For this review, use the dimensioned drawing (mm, ordinates from the lowest corner) and the shaded views. A direction names the side the tool comes from. Give positions to 0.01 mm unless a question says otherwise; leave off trailing zeros. Write each loop counter-clockwise with the first axis right and the second up, starting at its lowest first coordinate (ties: lowest second). Pieces come first, ordered by that corner, then holes. Notation, with made-up numbers: M -9.75,26.25 L 30.25,26.25 A31 cw 30.25,53.25 Z; hole C 8.5,53.5 d11. An arc over 180 degrees is marked long. Answer in a Markdown table with one row per item.
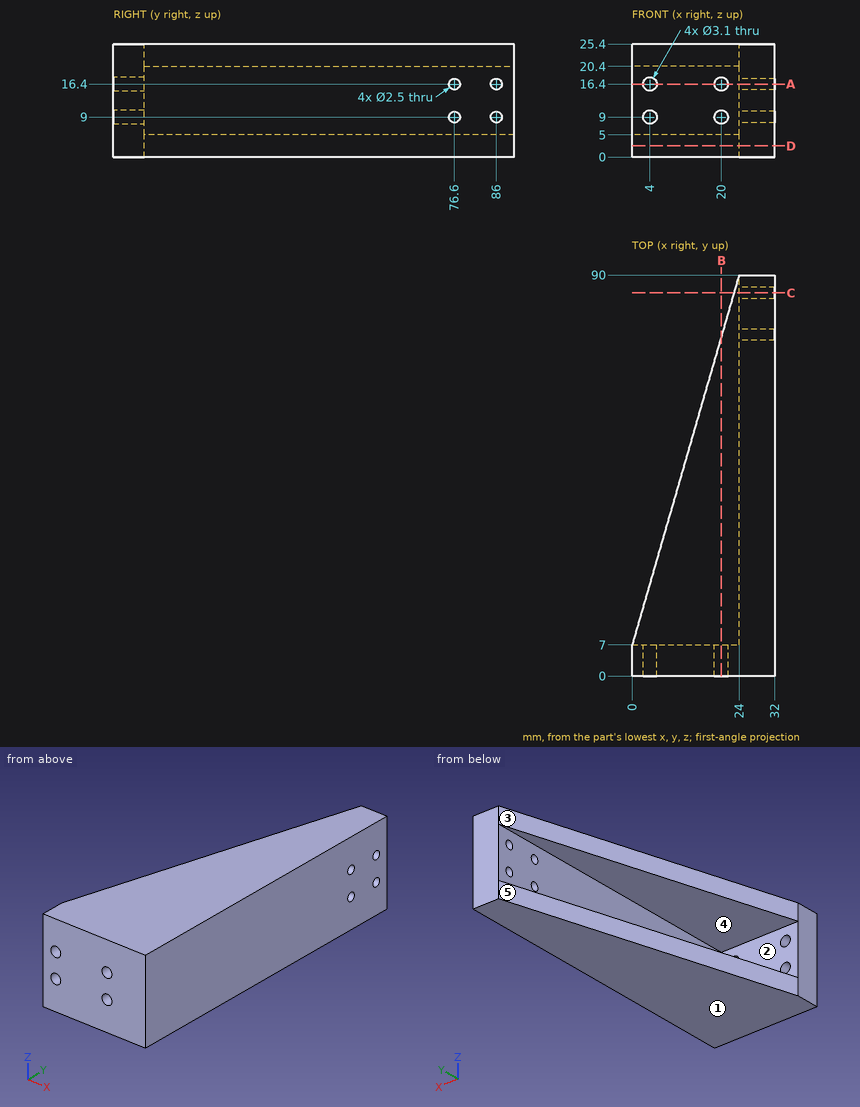
1) Add section A-A (z = 16.4). Write out the cut boundary in (x, y).
Geometry says:
| item | result |
|---|---|
| outline | M 0,0 L 2.45,0 L 2.45,7 L 0,7 Z; M 5.55,0 L 18.45,0 L 18.45,7 L 5.55,7 Z; M 21.55,0 L 32,0 L 32,75.35 L 24,75.35 L 24,7 L 21.55,7 Z; M 24,77.85 L 32,77.85 L 32,84.75 L 24,84.75 Z; M 24,87.25 L 32,87.25 L 32,90 L 24,90 Z |
2) The part is to be moulded in two halves that separate along Z. For the marked faces 1, 2 and 3, say which applies: released by +Z, released by -Z, zero draft, split by the parting line, or undercut.
Geometry says:
| item | result |
|---|---|
| face 1 | released by -Z |
| face 2 | undercut |
| face 3 | zero draft |
3) Add section B-B (x = 20). Write out the cut boundary in (y, z), and give its area (3 significant figures).
Geometry says:
| item | result |
|---|---|
| outline | M 0,0 L 76.17,0 L 76.17,5 L 7,5 L 7,7.45 L 0,7.45 Z; M 0,10.55 L 7,10.55 L 7,14.85 L 0,14.85 Z; M 0,17.95 L 7,17.95 L 7,20.4 L 76.17,20.4 L 76.17,25.4 L 0,25.4 Z |
| area | 826 mm^2 |
4) Add section D-D (z = 2.5). Write out the cut boundary in (x, y), and give its area (3 significant figures).
Geometry says:
| item | result |
|---|---|
| outline | M 0,0 L 32,0 L 32,90 L 24,90 L 0,7 Z |
| area | 1,880 mm^2 |
5) To check wall thickness, follow probe 1 along Y at (x, z) = (27.25, 9); probe 2 along Y at (x, z) = (26, 9.5); probe 3 along Z at (x, y) = (13, 23). State the ranges of each line that lie inside material, in increasing order. Write a range as [from, to].
Geometry says:
| item | result |
|---|---|
| probe 1 | [0, 75.35], [77.85, 84.75], [87.25, 90] |
| probe 2 | [0, 75.45], [77.75, 84.85], [87.15, 90] |
| probe 3 | [0, 5], [20.4, 25.4] |
6) For the marked faces 4 and 5, list the 3-axis set-ups (+Z, -Z, +X, -X, +Y, -Y) from which the entire face can be reached by the end or side of a thin tool; tool diameter is ignored.
Geometry says:
| item | result |
|---|---|
| face 4 | -X, +Y |
| face 5 | +Z, -Z, -X, +Y |
7) Insertion check: P1, Ø5, axis at x = 20.5, z = 10.5, coming from the +Y side; P2, Ø4, axis at y = 76.6, z = 16.4, coming from the -X side; P3, Ø2, axis at y = 86, z = 9, coming from the +X side; P4, Ø10, axis at y = 22, z = 7, coming from the -X side. Each pin has a flat end and moves straight along its axis. Give the tip position at first contact, or say it passes through.
Geometry says:
| item | result |
|---|---|
| P1 | y = 7 |
| P2 | x = 24 |
| P3 | through |
| P4 | x = 3.01 |
8) Add section C-C (y = 86). Write out the cut boundary in (x, z).
Geometry says:
| item | result |
|---|---|
| outline | M 22.84,0 L 32,0 L 32,7.75 L 24,7.75 L 24,5 L 22.84,5 Z; M 22.84,20.4 L 24,20.4 L 24,17.65 L 32,17.65 L 32,25.4 L 22.84,25.4 Z; M 24,10.25 L 32,10.25 L 32,15.15 L 24,15.15 Z |
